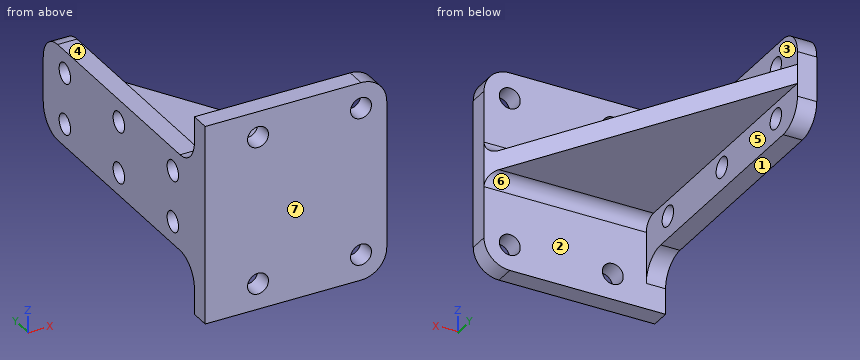
```python
from build123d import *

# Parameters (mm, degrees)
RESSALTO_EXTRUS_O1_DEPTH = 30
ESBO_O2_W                = 12
ESBO_O2_H                = 94
CORTE_EXTRUS_O1_DEPTH    = 118.541482039
ESBO_O3_W                = 30
ESBO_O3_H                = 10
CORTE_EXTRUS_O2_DEPTH    = 118.541482039
ESBO_O4_W                = 3.6
ESBO_O4_H                = 30
CORTE_EXTRUS_O3_DEPTH    = 108.498837203
ESBO_O5_W                = 56.4
ESBO_O5_H                = 6
RESSALTO_EXTRUS_O2_DEPTH = 16
ESBO_O6_W                = 56.4
ESBO_O6_H                = 6
RESSALTO_EXTRUS_O3_DEPTH = 16
FILETE1_R                = 8
FILETE2_R                = 8
FILETE3_R                = 8
FILETE4_R                = 4
ESBO_O7_R                = 3.175
CORTE_EXTRUS_O4_DEPTH    = 113.943171551
ESBO_O8_R                = 3.25
CORTE_EXTRUS_O5_DEPTH    = 112.143870726


with BuildPart() as part:
    # Esboço1 → Ressalto-extrusão1 (new body)
    with BuildSketch(Plane.XY):
        Polygon((0, 0), (0, 100), (60, 0), align=None)
    extrude(amount=RESSALTO_EXTRUS_O1_DEPTH)

    # Esboço2 → Corte-extrusão1 (cut, through all)
    with BuildSketch(Plane.ZY.offset(-6)):
        with Locations((24, 53)):
            Rectangle(ESBO_O2_W, ESBO_O2_H)
        with Locations((6, 53)):
            Rectangle(ESBO_O2_W, ESBO_O2_H)
    extrude(amount=-CORTE_EXTRUS_O1_DEPTH, mode=Mode.SUBTRACT)

    # Esboço3 → Corte-extrusão2 (cut, through all)
    with BuildSketch(Plane(origin=(6, 0, 0), x_dir=(0, 0, -1), z_dir=(1, 0, 0))):
        with Locations((-15, 95)):
            Rectangle(ESBO_O3_W, ESBO_O3_H)
    extrude(amount=-CORTE_EXTRUS_O2_DEPTH, mode=Mode.SUBTRACT)

    # Esboço4 → Corte-extrusão3 (cut, through all)
    with BuildSketch(Plane(origin=(0, 6, 0), x_dir=(1, 0, 0), z_dir=(0, 1, 0))):
        with Locations((58.2, -15)):
            Rectangle(ESBO_O4_W, ESBO_O4_H)
    extrude(amount=-CORTE_EXTRUS_O3_DEPTH, mode=Mode.SUBTRACT)

    # Esboço5 → Ressalto-extrusão2 (add)
    with BuildSketch(Plane.XY.offset(30)):
        with Locations((28.2, 3)):
            Rectangle(ESBO_O5_W, ESBO_O5_H)
    extrude(amount=RESSALTO_EXTRUS_O2_DEPTH)

    # Esboço6 → Ressalto-extrusão3 (add)
    with BuildSketch(Plane(origin=(0, 0, 0), x_dir=(-1, 0, 0), z_dir=(0, 0, -1))):
        with Locations((-28.2, 3)):
            Rectangle(ESBO_O6_W, ESBO_O6_H)
    extrude(amount=RESSALTO_EXTRUS_O3_DEPTH)

    # Filete1
    filete1_edges = [part.edges().sort_by_distance(p)[0] for p in [
        (3, 6, 0),
        (3, 6, 30),
    ]]
    fillet(filete1_edges, radius=FILETE1_R)

    # Filete2
    filete2_edges = [part.edges().sort_by_distance(p)[0] for p in [
        (56.4, 3, -16),
        (56.4, 3, 46),
    ]]
    fillet(filete2_edges, radius=FILETE2_R)

    # Filete3
    filete3_edges = [part.edges().sort_by_distance(p)[0] for p in [
        (3, 90, 30),
        (3, 90, 0),
    ]]
    fillet(filete3_edges, radius=FILETE3_R)

    # Filete4
    filete4_edges = [part.edges().sort_by_distance(p)[0] for p in [
        (31.2, 6, 18),
        (31.2, 6, 12),
    ]]
    fillet(filete4_edges, radius=FILETE4_R)

    # Esboço7 → Corte-extrusão4 (cut, through all)
    with BuildSketch(Plane(origin=(6, 0, 0), x_dir=(0, 0, -1), z_dir=(1, 0, 0))):
        with Locations((-23, 78)):
            Circle(ESBO_O7_R)
        with Locations((-23, 48)):
            Circle(ESBO_O7_R)
        with Locations((-23, 18)):
            Circle(ESBO_O7_R)
        with Locations(Location((-7, 18, 0), (0, 0, 180))):
            Circle(ESBO_O7_R)
        with Locations(Location((-7, 48, 0), (0, 0, 180))):
            Circle(ESBO_O7_R)
        with Locations(Location((-7, 78, 0), (0, 0, 180))):
            Circle(ESBO_O7_R)
    extrude(amount=-CORTE_EXTRUS_O4_DEPTH, mode=Mode.SUBTRACT)

    # Esboço8 → Corte-extrusão5 (cut, through all)
    with BuildSketch(Plane(origin=(0, 6, 0), x_dir=(1, 0, 0), z_dir=(0, 1, 0))):
        with Locations(Location((48.4, 8, 0), (0, 0, 270))):
            Circle(ESBO_O8_R)
        with Locations(Location((48.4, -38, 0), (0, 0, 270))):
            Circle(ESBO_O8_R)
        with Locations(Location((16.4, -38, 0), (0, 0, 270))):
            Circle(ESBO_O8_R)
        with Locations(Location((16.4, 8, 0), (0, 0, 270))):
            Circle(ESBO_O8_R)
    extrude(amount=-CORTE_EXTRUS_O5_DEPTH, mode=Mode.SUBTRACT)


solid = part.part
```
Could you check a few things on this model? Use its own coordinates, in mm. Face numbers are marked on the shaded views. A direction names the side the tool comes from. Give positions to 0.01 mm unless a question says otherwise; leave off trailing zeros. Loops run counter-clockwise (first coordinate to the right, second up) from the corner with the lowest first, then second, coordinate; pieces in that order, holes last. Notation, with made-up numbers: (30, -30) -> (48, -30) arc R34 ccw to (48, 5) -> close; hole circle Ø10 at (36.5, 56.25). An arc over 180 degrees is marked (long way). Put each result on its own line as item: value.
(1) Imagine slicing it at B-B on z = 23. Write out the boundary of the cut face in (x, y) (3 decimals), plus the area to 3 significant figures.
Computed:
outline: (0, 0) -> (56.4, 0) -> (56.4, 6) -> (6, 6) -> (6, 14.825) -> (0, 14.825) -> close; (0, 21.175) -> (6, 21.175) -> (6, 44.825) -> (0, 44.825) -> close; (0, 51.175) -> (6, 51.175) -> (6, 74.825) -> (0, 74.825) -> close; (0, 81.175) -> (6, 81.175) -> (6, 89.937) -> (0, 89.937) -> close
area: 728 mm^2
(2) Thinking about a two-plate mould opening in Y: for the marked faces 5, 6 and 7, which applies, pulls with the +Y half, pulls with the -Y half, needs draft (parallel to the pull), parting line crosses it, or undercut?
Computed:
face 5: needs draft
face 6: pulls with the +Y half
face 7: pulls with the -Y half
(3) Imagine slicing it at C-C on y = 40.5. Write out the boundary of the cut face in (x, z).
Computed:
outline: (0, 0) -> (6, 0) -> (6, 12) -> (35.7, 12) -> (35.7, 18) -> (6, 18) -> (6, 30) -> (0, 30) -> close
(4) I'm going to push flat-ended pins straight in: pin 1 Ø4 at (x, z) = (50.5, -5.5) entering from +Y; pin 2 Ø4 at (y, z) = (78, 23) entering from -X; pin 3 Ø6 at (y, z) = (73.5, 30.5) entering from +X; pin 4 Ø4 at (x, y) = (25, 37.5) entering from -Z. Where does each tip first touch, or does it pass through?
Computed:
pin 1: y = 6
pin 2: through
pin 3: x = 6
pin 4: z = 12
(5) Please list where these lines run through material, in increasing order: probe 1 along Y at (x, z) = (4.5, 23) (3 decimals); probe 2 along X at (y, z) = (21, 3.5). Write a range as [from, to].
Computed:
probe 1: [0, 14.825], [21.175, 44.825], [51.175, 74.825], [81.175, 89.937]
probe 2: [0, 6]
(6) For the marked faces 1, 2, 3 and 4, which set-ups out of +Z, -Z, +X, -X, +Y, -Y let a thin tool reach every point of the face, with its end or its side?
Computed:
face 1: -Z, +X, -X, +Y
face 2: -Z, +X, +Y
face 3: +Z, +X, +Y
face 4: +Z, +X, -X, +Y
(7) Imagine slicing it at A-A on y = 78. Write out the boundary of the cut face in (x, z) (3 decimals).
Computed:
outline: (0, 0) -> (6, 0) -> (6, 3.825) -> (0, 3.825) -> close; (0, 10.175) -> (6, 10.175) -> (6, 12) -> (13.2, 12) -> (13.2, 18) -> (6, 18) -> (6, 19.825) -> (0, 19.825) -> close; (0, 26.175) -> (6, 26.175) -> (6, 30) -> (0, 30) -> close
(8) Imagine slicing it at D-D on x = 16.4. Write out the boundary of the cut face in (y, z), plus the area to 3 significant figures.
Computed:
outline: (0, -16) -> (6, -16) -> (6, -11.25) -> (0, -11.25) -> close; (0, -4.75) -> (6, -4.75) -> (6, 8) arc R4 cw to (10, 12) -> (72.67, 12) -> (72.67, 18) -> (10, 18) arc R4 cw to (6, 22) -> (6, 34.75) -> (0, 34.75) -> close; (0, 41.25) -> (6, 41.25) -> (6, 46) -> (0, 46) -> close
area: 701 mm^2
